from build123d import *

# Parameters (mm, degrees)
SKETCH1_R             = 1.5748
BOSS_EXTRUDE1_DEPTH   = 1.27
BOSS_EXTRUDE1_2_DEPTH = 1.27
BOSS_EXTRUDE2_DEPTH   = 1.27
SKETCH3_R             = 0.8255
CUT_EXTRUDE1_DEPTH    = 5.08


with BuildPart() as part:
    # Sketch1 → Boss-Extrude1 (new, symmetric)
    with BuildSketch(Plane.XY):
        with Locations((3.175, 0)):
            Circle(SKETCH1_R)
    extrude(amount=BOSS_EXTRUDE1_DEPTH, both=True)



with BuildPart() as body_2:
    # Sketch1 → Boss-Extrude1 2 (new, symmetric)
    with BuildSketch(Plane.XY):
        with Locations((-3.175, 0)):
            Circle(SKETCH1_R)
    extrude(amount=BOSS_EXTRUDE1_2_DEPTH, both=True)


with BuildPart() as part_1:
    add(part.part)

    add(body_2.part)  # Boss-Extrude2 merges body 2
    # Sketch2 → Boss-Extrude2 (add)
    with BuildSketch(Plane.XY.offset(1.27)):
        with BuildLine():
            ThreePointArc((1.5875, -1.982786864), (5.715, 0), (1.5875, 1.982786864))
            ThreePointArc((1.5875, 1.982786864), (0, 1.425573729), (-1.5875, 1.982786864))
            ThreePointArc((-1.5875, 1.982786864), (-5.715, 0), (-1.5875, -1.982786864))
            ThreePointArc((-1.5875, -1.982786864), (0, -1.425573729), (1.5875, -1.982786864))
        make_face()
    boss_extrude2 = extrude(amount=BOSS_EXTRUDE2_DEPTH)

    # Mirror1: Boss-Extrude2 across plane
    add(boss_extrude2.mirror(Plane.XY))

    # Sketch3 → Cut-Extrude1 (cut)
    with BuildSketch(Plane.XY.offset(2.54)):
        with Locations((3.175, 0)):
            Circle(SKETCH3_R)
        with Locations((-3.175, 0)):
            Circle(SKETCH3_R)
    extrude(amount=-CUT_EXTRUDE1_DEPTH, mode=Mode.SUBTRACT)


solid = part_1.part
Input: part model. Units: mm. Frame: model coordinates. A direction names the side the tool comes from. Give positions to 0.01 mm unless a question says otherwise; leave off trailing zeros. Loops run counter-clockwise (first coordinate to the right, second up) from the corner with the lowest first, then second, coordinate; pieces in that order, holes last. Notation, with made-up numbers: (-32, 74.25) -> (-12, 74.25) arc R7 cw to (-12, 78.25) -> close; hole circle Ø11 at (0.25, 51). An arc over 180 degrees is marked (long way). Answer as a JSON object with one key per item and string values. Group by question number.
Item 1: Cut plane B-B, the plane z = -0.85. Return the cut outline in (x, y) (1 decimal), and give its area (3 significant figures).
Item 2: Cut plane C-C, the plane x = 3.25. Return the cut outline in (y, z), and give its area (3 significant figures).
Item 3: Pin query (flat end, axial travel): P1, Ø2.5, axis at x = 3.175, y = 0, coming from the +Z side; P2, Ø1.5, axis at x = -3.175, y = 0, coming from the -Z side. Return the tip coordinate at first contact, or that it passes through.
Item 4: Pull-direction query (X, two-part tool) for faces 1 (the flat face through (0, 0, -2.54)), 2 (the cylindrical face through (4.63, -0.6, 0.02)); classes: released by +X, released by -X, zero draft, split by the parting line, or undercut.
Item 5: Cut plane D-D, the plane y = -1. Return the cut outline in (x, z), and give its area (3 significant figures).
Item 6: Reachability of faces 3 (the cylindrical face through (4, 0, 0)), 4 (the flat face through (0, 0, -1.27)) from +Z, -Z, +X, -X, +Y, -Y: full face, straight path, thin tool, end or side. Return the list, or none.
Item 7: Line query: probe 1 along Z at (x, y) = (-2.5, 2.3); probe 2 along X at (y, z) = (0.25, 2.15); probe 3 along Y at (x, z) = (-2.75, -1). Output: solid intervals per line, ascending.
Item 8: Cut plane A-A, the plane y = 0. Return the cut outline in (x, z) (1 decimal).
Checks:
{
 "1": {"outline": "circle Ø3.1 at (-3.2, 0); circle Ø3.1 at (3.2, 0); hole circle Ø1.7 at (-3.2, 0); hole circle Ø1.7 at (3.2, 0)", "area": "11.3 mm²"},
 "2": {"outline": "(-2.54, -2.54) -> (-0.82, -2.54) -> (-0.82, 2.54) -> (-2.54, 2.54) -> (-2.54, 1.27) -> (-1.57, 1.27) -> (-1.57, -1.27) -> (-2.54, -1.27) -> close; (0.82, -2.54) -> (2.54, -2.54) -> (2.54, -1.27) -> (1.57, -1.27) -> (1.57, 1.27) -> (2.54, 1.27) -> (2.54, 2.54) -> (0.82, 2.54) -> close", "area": "12.5 mm²"},
 "3": {"P1": "stops at z = 2.54", "P2": "passes through"},
 "4": {"face 1": "zero draft", "face 2": "undercut"},
 "5": {"outline": "(-5.51, -2.54) -> (5.51, -2.54) -> (5.51, -1.27) -> (4.39, -1.27) -> (4.39, 1.27) -> (5.51, 1.27) -> (5.51, 2.54) -> (-5.51, 2.54) -> (-5.51, 1.27) -> (-4.39, 1.27) -> (-4.39, -1.27) -> (-5.51, -1.27) -> close; hole (-1.96, -1.27) -> (1.96, -1.27) -> (1.96, 1.27) -> (-1.96, 1.27) -> close", "area": "40.4 mm²"},
 "6": {"face 3": "+Z, -Z", "face 4": "none"},
 "7": {"probe 1": "z = -2.54 to -1.27, 1.27 to 2.54", "probe 2": "x = -5.7 to -3.96, -2.39 to 2.39, 3.96 to 5.7", "probe 3": "y = -1.52 to -0.71, 0.71 to 1.52"},
 "8": {"outline": "(-5.7, -2.5) -> (-4, -2.5) -> (-4, 2.5) -> (-5.7, 2.5) -> (-5.7, 1.3) -> (-4.7, 1.3) -> (-4.7, -1.3) -> (-5.7, -1.3) -> close; (-2.3, -2.5) -> (2.3, -2.5) -> (2.3, 2.5) -> (-2.3, 2.5) -> close; (4, -2.5) -> (5.7, -2.5) -> (5.7, -1.3) -> (4.7, -1.3) -> (4.7, 1.3) -> (5.7, 1.3) -> (5.7, 2.5) -> (4, 2.5) -> close; hole (-1.6, -1.3) -> (1.6, -1.3) -> (1.6, 1.3) -> (-1.6, 1.3) -> close"}
}
